Verification items for the finished model (mm, model axes). A direction names the side the tool comes from. Round coordinates to 2 decimals unless told otherwise and drop trailing zeros. Order: outer loops, then holes, each group sorted by start corner. A loop starts at its lowest first (then second) coordinate and runs counter-clockwise, first axis right, second up. Notation, with made-up numbers: M 69.25,73 L 116.25,73 A37 ccw 116.25,112 Z; hole C 5,26.25 d8. An arc over 180 degrees is marked long. Use one line per item in the form item = value. Start each with the question number.
Item 1: Cross-section at B-B on x = 11.5. Enter the section's corners in (y, z), then the cut area to 3 significant figures.
Item 2: Thickness scan on probe 1 along Y at (x, z) = (3.5, 3); probe 2 along X at (y, z) = (15.25, 20); probe 3 along Y at (x, z) = (15, 6.75). Record the ranges inside material, lowest first. Write a range as [from, to].
Item 3: Cross-section at A-A on z = 10.75. Enter the section's corners in (x, y).
Item 4: Cross-section at C-C on x = 3.25. Enter the section's corners in (y, z).
Item 5: Release check for a two-part mould opening along Y. For faces 1 (the cylindrical face through (3.305, 27.987, 4.056)), 2 (the flat face through (10, 20, 26)), 3 (the flat face through (21.5, 15, 17)), 4 (the flat face through (15, 0, 4)) record: +Y half, -Y half, draft (parallel to the pull), parting line (faces both ways), or undercut.
Item 6: Cross-section at D-D on y = 8. Enter the section's corners in (x, z).
Item 7: Go/stop test with flat-tipped pins: pin 1 Ø2.5 at (y, z) = (14, 13.5) entering from -X; pin 2 Ø1.5 at (x, z) = (23.5, 21.5) entering from +Y; pin 3 Ø2.5 at (y, z) = (13, 14.5) entering from +X. Record where each tip stops, or that it passes through.
Item 8: Tool access check on faces 5 (the flat face through (8, 15, 0)), 6 (the flat face through (18.2, 9.34, 16.87)). Record the directions out of +Z, -Z, +X, -X, +Y, -Y that give a thin tool (end or side, any length) a straight path to the whole face; none if there is none.
from build123d import *

# Parameters (mm, degrees)
IZIM1_W                     = 30
IZIM1_H                     = 30
Y_KSEKLIK_EKSTR_ZYON1_DEPTH = 8
IZIM2_R                     = 12.5
Y_KSEKLIK_EKSTR_ZYON2_DEPTH = 8
IZIM3_R                     = 5.5
KES_EKSTR_ZYON1_DEPTH       = 8
IZIM4_R                     = 1.5
KES_EKSTR_ZYON2_DEPTH       = 8
IZIM5_R                     = 12.5
Y_KSEKLIK_EKSTR_ZYON3_DEPTH = 10


with BuildPart() as part:
    # Çizim1 → Yükseklik-Ekstrüzyon1 (new body)
    with BuildSketch(Plane.XY):
        with Locations((15, 15)):
            Rectangle(IZIM1_W, IZIM1_H)
    extrude(amount=Y_KSEKLIK_EKSTR_ZYON1_DEPTH)

    # Çizim2 → Yükseklik-Ekstrüzyon2 (add)
    with BuildSketch(Plane.XY.offset(8)):
        with Locations(Location((15, 15, 0), (0, 0, 180))):
            Circle(IZIM2_R)
        Polygon((15, 22.505553499), (8.5, 18.75277675), (8.5, 11.24722325), (15, 7.494446501), (21.5, 11.24722325), (21.5, 18.75277675), align=None, mode=Mode.SUBTRACT)
    extrude(amount=Y_KSEKLIK_EKSTR_ZYON2_DEPTH)

    # Çizim3 → Kes-Ekstrüzyon1 (cut)
    with BuildSketch(Plane.XY.offset(8)):
        with Locations((15, 15)):
            Circle(IZIM3_R)
    extrude(amount=-KES_EKSTR_ZYON1_DEPTH, mode=Mode.SUBTRACT)

    # Çizim4 → Kes-Ekstrüzyon2 (cut)
    with BuildSketch(Plane.XY.offset(8)):
        with Locations((3.5, 26.5)):
            Circle(IZIM4_R)
        with Locations((26.5, 26.5)):
            Circle(IZIM4_R)
        with Locations((26.5, 3.5)):
            Circle(IZIM4_R)
        with Locations((3.5, 3.5)):
            Circle(IZIM4_R)
    extrude(amount=-KES_EKSTR_ZYON2_DEPTH, mode=Mode.SUBTRACT)

    # Çizim5 → Yükseklik-Ekstrüzyon3 (add)
    with BuildSketch(Plane.XY.offset(16)):
        with Locations(Location((15, 15, 0), (0, 0, 180))):
            Circle(IZIM5_R)
        Polygon((15, 22.505553499), (8.5, 18.75277675), (8.5, 11.24722325), (15, 7.494446501), (21.5, 11.24722325), (21.5, 18.75277675), align=None, mode=Mode.SUBTRACT)
    extrude(amount=Y_KSEKLIK_EKSTR_ZYON3_DEPTH)


solid = part.part
Output values:
q1.outline = M 0,0 L 10.76,0 L 10.76,8 L 9.52,8 L 9.52,26 L 3,26 L 3,8 L 0,8 Z; M 19.24,0 L 30,0 L 30,8 L 27,8 L 27,26 L 20.48,26 L 20.48,8 L 19.24,8 Z
q1.area = 407 mm2
q2.probe_1 = [0, 2], [5, 25], [28, 30]
q2.probe_2 = [2.5, 8.5], [21.5, 27.5]
q2.probe_3 = [0, 9.5], [20.5, 30]
q3.outline = C 15,15 d25; hole M 8.5,11.25 L 15,7.49 L 21.5,11.25 L 21.5,18.75 L 15,22.51 L 8.5,18.75 Z
q4.outline = M 0,0 L 2.02,0 L 2.02,8 L 0,8 Z; M 4.98,0 L 25.02,0 L 25.02,8 L 19.26,8 L 19.26,26 L 10.74,26 L 10.74,8 L 4.98,8 Z; M 27.98,0 L 30,0 L 30,8 L 27.98,8 Z
q5.face_1 = undercut
q5.face_2 = draft
q5.face_3 = undercut
q5.face_4 = -Y half
q6.outline = M 0,0 L 30,0 L 30,8 L 25.36,8 L 25.36,26 L 15.88,26 L 15.88,8 L 14.12,8 L 14.12,26 L 4.64,26 L 4.64,8 L 0,8 Z
q7.pin_1 = 2.5
q7.pin_2 = 24.81
q7.pin_3 = 27.48
q8.face_5 = -Z, +X, -X, +Y, -Y
q8.face_6 = +Z
